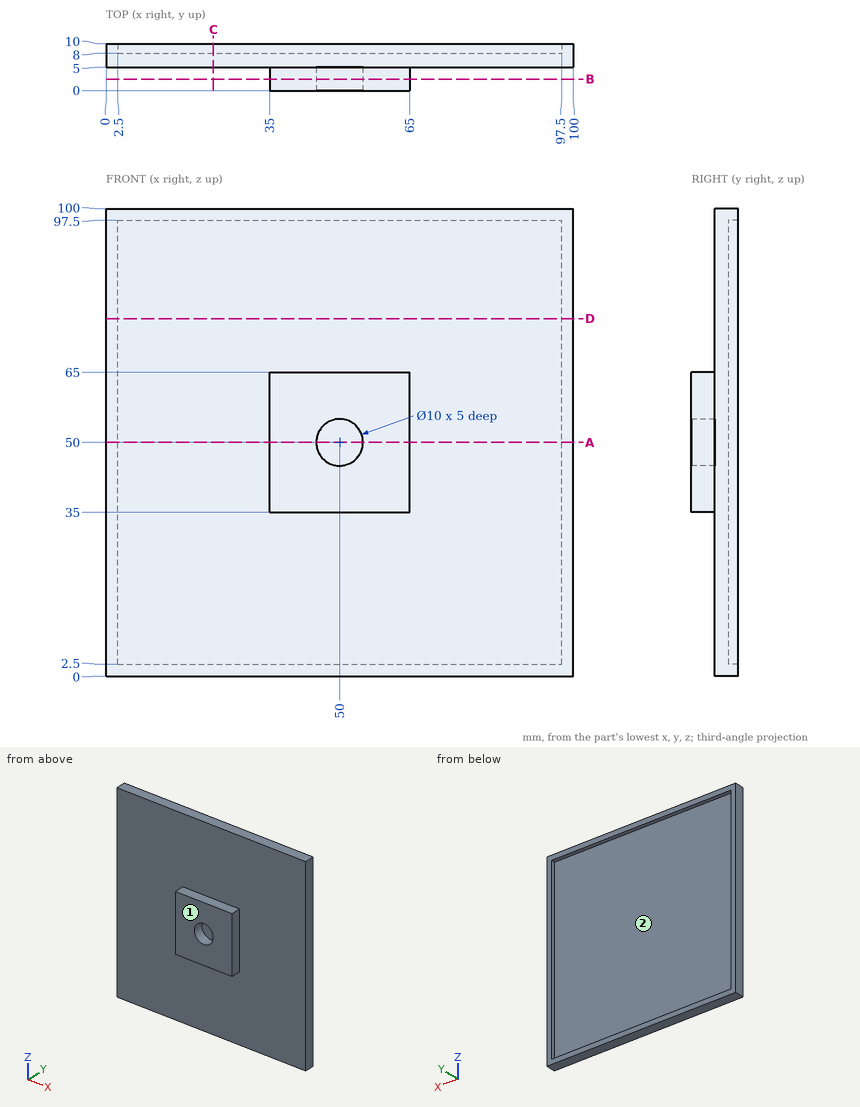
Verification items for this drawing (mm, ordinates from the low corner). Coordinates: 2 decimals unless noted, no trailing zeros. Loops run counter-clockwise (first coordinate to the right, second up) from the corner with the lowest first, then second, coordinate; pieces in that order, holes last. Notation, with made-up numbers: (60, 20) -> (110, 20) arc R25 cw to (110, 51) -> close; hole circle Ø2 at (-28, 72.5). An arc over 180 degrees is marked (long way). Answer in a Markdown table with one row per item. Add a question column.
1. Material ranges on probe 1 along Z at (x, y) = (14.5, 8.25); probe 2 along Z at (x, y) = (50, 1.55); probe 3 along Y at (x, z) = (59, 92), recorded low to high. Write a range as [from, to].
2. Section check D-D, the plane z = 76.5. Enter the section's corners in (x, y).
3. Section check C-C, the plane x = 23. Enter the section's corners in (y, z), then the cut area to 3 significant figures.
4. Section check B-B, the plane y = 2.5. Enter the section's corners in (x, z), then the cut area to 3 significant figures.
5. Section check A-A, the plane z = 50. Enter the section's corners in (x, y), then the cut area to 3 significant figures.
6. Depth check by flat-ended pin: P1, Ø1, axis at y = 8.5, z = 30.5, coming from the -X side; P2, Ø2.5, axis at y = 1.5, z = 45.5, coming from the -X side; P3, Ø6, axis at x = 50, z = 50, coming from the -Y side; P4, Ø4, axis at x = 62.5, y = 1.5, coming from the -Z side. Enter the tip coordinate at first touch or a pass-through.
7. Draft check along Y on the marked faces 1 and 2. Enter one of: +Y half, -Y half, draft (parallel to the pull), parting line (faces both ways), or undercut.
Derived:
| question | item | result |
|---|---|---|
| 1 | probe 1 | z = [0, 2.5], [97.5, 100] |
| 1 | probe 2 | z = [35, 45], [55, 65] |
| 1 | probe 3 | y = [5, 8] |
| 2 | outline | (0, 5) -> (100, 5) -> (100, 10) -> (97.5, 10) -> (97.5, 8) -> (2.5, 8) -> (2.5, 10) -> (0, 10) -> close |
| 3 | outline | (5, 0) -> (10, 0) -> (10, 2.5) -> (8, 2.5) -> (8, 97.5) -> (10, 97.5) -> (10, 100) -> (5, 100) -> close |
| 3 | area | 310 mm² |
| 4 | outline | (35, 35) -> (65, 35) -> (65, 65) -> (35, 65) -> close; hole circle Ø10 at (50, 50) |
| 4 | area | 821 mm² |
| 5 | outline | (0, 5) -> (35, 5) -> (35, 0) -> (45, 0) -> (45, 5) -> (55, 5) -> (55, 0) -> (65, 0) -> (65, 5) -> (100, 5) -> (100, 10) -> (97.5, 10) -> (97.5, 8) -> (2.5, 8) -> (2.5, 10) -> (0, 10) -> close |
| 5 | area | 410 mm² |
| 6 | P1 | stops at x = 0 |
| 6 | P2 | stops at x = 35 |
| 6 | P3 | stops at y = 5 |
| 6 | P4 | stops at z = 35 |
| 7 | face 1 | -Y half |
| 7 | face 2 | +Y half |
